Could you check a few things on this model? Use its own coordinates, in mm. A direction names the side the tool comes from. Coordinates: 2 decimals unless noted, no trailing zeros. Loops run counter-clockwise (first coordinate to the right, second up) from the corner with the lowest first, then second, coordinate; pieces in that order, holes last. Notation, with made-up numbers: (44, 51.5) -> (73, 51.5) arc R17 ccw to (73, 69.5) -> close; hole circle Ø2 at (73.5, -15.5). An arc over 180 degrees is marked (long way). One line per question, with ' | ' between items.
Autodesk Inventor part; units mm, degrees
ref_plane "YZ Plane" through (0, 0, 0) normal (1, 0, 0) x (0, 1, 0)
ref_plane "XZ Plane" through (0, 0, 0) normal (0, 1, 0) x (-1, 0, 0)
ref_plane "XY Plane" through (0, 0, 0) normal (0, 0, 1) x (1, 0, 0)
sketch "Sketch1" plane through (0, 0, 0) normal (0, 0, 1) x (1, 0, 0)
  line L0 (0, 0) -> (-50.8, 0)
  line L1 (-50.8, 0) -> (-50.8, -101.6)
  line L2 (-50.8, -101.6) -> (0, -101.6)
  line L3 (0, -22.225) -> (-38.1, -22.225)
  line L4 (-38.1, -22.225) -> (-38.1, -41.275)
  line L5 (-38.1, -41.275) -> (0, -41.275)
  line L6 (0, -101.6) -> (0, -41.275)
  line L7 (0, -22.225) -> (0, 0)
  dimension "d0" = 101.6
  dimension "d1" = 50.8
  dimension "d4" = 22.225
  dimension "d5" = 38.1
  dimension "d6" = 19.05
extrude "Extrusion1" add sketch "Sketch1" along normal blind 31.75
sketch "Sketch2" plane through (0, -22.225, 0) normal (1, 0, 0) x (0, 0, -1)
  line L0 (-31.75, 0) -> (-31.75, 22.225)
  line L1 (0, 22.225) -> (0, -79.375)
  line L2 (-31.75, 22.225) -> (0, 22.225)
  line L3 (0, 22.225) -> (0, -79.375)
  line L4 (0, -79.375) -> (-31.75, -79.375)
  line L5 (-31.75, -79.375) -> (-31.75, 22.225)
extrude "Extrusion2" cut sketch "Sketch2" against normal blind 0.381
sketch "Sketch3" plane through (-50.8, 0, 31.75) normal (0, 1, 0) x (1, 0, 0)
  line L0 (0, 31.75) -> (0, 0)
  line L1 (50.419, 31.75) -> (0, 31.75)
  point P0 (50.8, 31.75)
  point P1 (38.1, 15.875)
  dimension "d9" = 38.1
  dimension "d10" = 15.875
hole "Hole1" at (-12.7, 0, 15.875) direction (0, -1, 0) diameter 6.7564 end up to surface
sketch "Sketch4" plane through (-50.8, -101.6, 0) normal (-1, 0, 0) x (0, 0, 1)
  line L0 (0, 101.6) -> (0, 0)
  line L1 (0, 101.6) -> (31.75, 101.6)
  point P0 (15.875, 69.85)
  dimension "d18" = 15.875
  dimension "d19" = 31.75
hole "Hole2" at (-50.8, -31.75, 15.875) direction (1, 0, 0) diameter 6.7564 end through all
sketch "Sketch5" plane through (-50.8, -101.6, 0) normal (-1, 0, 0) x (0, 0, 1)
  line L0 (0, 101.6) -> (0, 0)
  line L1 (0, 101.6) -> (31.75, 101.6)
  point P0 (15.875, 31.75)
  dimension "d27" = 15.875
  dimension "d28" = 69.85
hole "Hole3" at (-50.8, -69.85, 15.875) direction (1, 0, 0) diameter 19.558 end through all
sketch "Sketch6" plane through (0, 0, 31.75) normal (0, 0, 1) x (1, 0, 0)
  line L0 (-0.381, 0) -> (-50.8, 0)
  line L1 (-50.8, 0) -> (-50.8, -101.6)
  point P0 (0, 0)
  point P1 (-25.4, -69.85)
  dimension "d36" = 69.85
  dimension "d37" = 25.4
hole "Hole4" at (-25.4, -69.85, 31.75) direction (0, 0, -1) diameter 6.7564 end through all
sketch "Sketch7" plane through (0, 0, 31.75) normal (0, 0, 1) x (1, 0, 0)
  circle A0 centre (-25.4, -107.95) radius 20.32
  line L0 (-0.381, 0) -> (-50.8, 0)
  line L1 (-50.8, 0) -> (-50.8, -101.6)
  point P0 (0, 0)
  dimension "d45" = 107.95
  dimension "d46" = 25.4
  dimension "d47" = 40.64
extrude "Extrusion3" cut sketch "Sketch7" against normal through all
properties part number "Over Support For Arm With Delrin"
Q1. We'd pull the mould along X, two halves only. Please class faces 1 (the face through (-50.8, -50, 16)), 2 (the face through (-25.044, -87.633, 16.097)), 3 (the face through (-25.549, -66.475, 3.302)), 4 (the face through (-19, -22.225, 16)): released by +X, released by -X, zero draft, split by the parting line, or undercut.
Values follow:
face 1: released by -X | face 2: undercut | face 3: undercut | face 4: zero draft
Q2. Please list where these lines run through material, in increasing order: L1, parallel to Y at x = -3, z = 27.5 (3 decimals); L2, parallel to Z at x = -5.5, y = -70; L3, parallel to X at y = -69.85, z = 26.75. Write a range as [from, to].
Values follow:
L1: y = [-101.6, -41.275], [-22.225, 0] | L2: z = [0, 6.1], [25.65, 31.75] | L3: x = [-50.8, -28.78], [-22.02, -0.38]
Q3. Imagine slicing it at B-B on x = -25.4. Write out the boundary of the cut face in (y, z) (3 decimals), plus the area to 3 significant figures.
Values follow:
outline: (-87.63, 0) -> (-73.228, 0) -> (-73.228, 6.698) arc R9.779 cw to (-73.228, 25.052) -> (-73.228, 31.75) -> (-87.63, 31.75) -> close; (-66.472, 0) -> (-41.275, 0) -> (-41.275, 31.75) -> (-66.472, 31.75) -> (-66.472, 25.052) arc R9.779 cw to (-66.472, 6.698) -> close; (-22.225, 0) -> (0, 0) -> (0, 31.75) -> (-22.225, 31.75) -> close | area: 1,790 mm2
Q4. For pin 1 (6 mm diameter, centred on x = -25.4, y = -69.85, fed in from +Z); pin 2 (1.5 mm diameter, centred on x = -15.5, z = 6, fed in from -Y); pin 3 (6 mm diameter, centred on x = -25.5, z = 18, fed in from -Y); pin 4 (9.5 mm diameter, centred on x = -24.5, z = 17.5, fed in from -Y), each with a flat end and sliding along its axis, tell me the tip position at first contact or that it passes through.
Values follow:
pin 1: passes through | pin 2: stops at y = -90.64 | pin 3: stops at y = -87.87 | pin 4: stops at y = -88.43
Q5. Imagine slicing it at A-A on y = -69.85. Write out the boundary of the cut face in (x, z), plus the area to 3 significant figures.
Values follow:
outline: (-50.8, 0) -> (-28.78, 0) -> (-28.78, 6.1) -> (-50.8, 6.1) -> close; (-50.8, 25.65) -> (-28.78, 25.65) -> (-28.78, 31.75) -> (-50.8, 31.75) -> close; (-22.02, 0) -> (-0.38, 0) -> (-0.38, 6.1) -> (-22.02, 6.1) -> close; (-22.02, 25.65) -> (-0.38, 25.65) -> (-0.38, 31.75) -> (-22.02, 31.75) -> close | area: 532 mm2
Q6. Imagine slicing it at C-C on z = 4.5. Write out the boundary of the cut face in (x, y) (3 decimals).
Values follow:
outline: (-50.8, -101.6) -> (-44.702, -101.6) arc R20.32 cw to (-6.098, -101.6) -> (-0.381, -101.6) -> (-0.381, -41.275) -> (-38.1, -41.275) -> (-38.1, -22.225) -> (-0.381, -22.225) -> (-0.381, 0) -> (-50.8, 0) -> close; hole circle Ø6.756 at (-25.4, -69.85)
Q7. For faces 5 (the face through (-20, -41.275, 16)), 6 (the face through (-0.381, -78, 23)), 7 (the face through (-11.406, -11.268, 18.996)), which set-ups out of +Z, -Z, +X, -X, +Y, -Y let a thin tool reach every point of the face, with its end or its side?
Values follow:
face 5: +Z, -Z, +X | face 6: +Z, -Z, +X, +Y, -Y | face 7: +Y
Q8. Imagine slicing it at D-D on y = -31.75. Write out the boundary of the cut face in (x, z).
Values follow:
outline: (-50.8, 0) -> (-38.1, 0) -> (-38.1, 12.5) -> (-50.8, 12.5) -> close; (-50.8, 19.25) -> (-38.1, 19.25) -> (-38.1, 31.75) -> (-50.8, 31.75) -> close
